```python
from build123d import *

# Parameters (mm, degrees)
SKETCH1_R           = 2.54
SKETCH1_R_2         = 2.25
BOSS_EXTRUDE1_DEPTH = 1.5875


with BuildPart() as part:
    # Sketch1 → Boss-Extrude1 (new body)
    with BuildSketch(Plane.XY):
        with BuildLine():
            Line((0, 0), (-44.45, 0))
            ThreePointArc((-44.45, 0), (-49.830627072, 1.070273269), (-54.392102448, 4.118153673))
            Line((-54.392102448, 4.118153673), (-86.142102448, 35.868153673))
            ThreePointArc((-86.142102448, 35.868153673), (-88.614208366, 37.519962038), (-91.530256121, 38.1))
            Line((-91.530256121, 38.1), (-99.06, 38.1))
            ThreePointArc((-99.06, 38.1), (-102.652102448, 36.612102448), (-104.14, 33.02))
            Line((-104.14, 33.02), (-104.14, 11.43))
            ThreePointArc((-104.14, 11.43), (-102.652102448, 7.837897552), (-99.06, 6.35))
            Line((-99.06, 6.35), (-99.06, -19.05))
            ThreePointArc((-99.06, -19.05), (-102.741703947, -21.834795846), (-104.14, -26.234204897))
            Line((-104.14, -26.234204897), (-104.14, -43.199318572))
            ThreePointArc((-104.14, -43.199318572), (-99.814124397, -51.831543955), (-90.309725681, -53.532990354))
            Line((-90.309725681, -53.532990354), (-38.1, -38.1))
            Line((-38.1, -38.1), (0, -38.1))
            Line((0, -38.1), (0, 0))
        make_face()
        with Locations((-89, 25.555)):
            Circle(SKETCH1_R, mode=Mode.SUBTRACT)
        with Locations((-89, -45.055)):
            Circle(SKETCH1_R, mode=Mode.SUBTRACT)
        with Locations((-18.24, -9.75)):
            Circle(SKETCH1_R, mode=Mode.SUBTRACT)
        with Locations((-74.5, -9.75)):
            Circle(SKETCH1_R_2, mode=Mode.SUBTRACT)
        with Locations((-48.5, -9.75)):
            Circle(SKETCH1_R_2, mode=Mode.SUBTRACT)
    extrude(amount=BOSS_EXTRUDE1_DEPTH)


solid = part.part
```
Build history of the part. All positions in model axes, mm. A direction names the side the tool comes from. Coordinates: 2 decimals unless noted, no trailing zeros. Order: outer loops, then holes, each group sorted by start corner. A loop starts at its lowest first (then second) coordinate and runs counter-clockwise, first axis right, second up. Notation, with made-up numbers: (-30.5, 0) -> (-15.5, 0) arc R32 ccw to (-15.5, 27) -> close; hole circle Ø5 at (4.5, 22). An arc over 180 degrees is marked (long way). Answer in a Markdown table with one row per item. Add a question column.
Q1. Drop flat-ended pins along their axis: pin 1 (3.5 mm diameter, centred on x = -74.5, y = -9.75, fed in from +Z); pin 2 (0.8 mm diameter, centred on x = -27, z = 1, fed in from +Y); pin 3 (0.5 mm diameter, centred on y = -11.5, z = 1, fed in from -X). Give the stop position or say it passes through.
Q2. Band-saw the part on A-A, the plane x = -89. List the corners of the cut face in (y, z) (1 decimal), then the cut area to 3 significant figures.
Q3. Mould opens along Y. For faces 3 (the face through (-88.576, 37.504, 0.783)), 4 (the face through (-17.068, -12.003, 0.783)), 5 (the face through (-64, -18, 0)) say: +Y half, -Y half, draft (parallel to the pull), parting line (faces both ways), or undercut.
Q4. Wall check: line 1 along Y through (x, z) = (-35, 0.15); line 2 along Y through (x, z) = (-48.5, 0.55); line 3 along Y through (x, z) = (-18.24, 0.75). Give the ranges that are in metal, low to high. Write a range as [from, to].
Q5. Band-saw the part on C-C, the plane x = -18.24. List the corners of the cut face in (y, z).
Q6. Which spindle directions (+Z, -Z, +X, -X, +Y, -Y) get a long thin tool onto all of the face, cutting with end or side? Do faces 1 (the face through (-102.612, 36.651, 0.783)), 2 (the face through (-102.691, 7.878, 0.783)). Say none if no direction does.
Q7. Band-saw the part on B-B, the plane y = -9.75. List the corners of the cut face in (x, z).
Q8. Band-saw the part on D-D, the plane z = 1.05. List the corners of the cut face in (x, y) (3 decimals).
Answers follow:
| question | item | result |
|---|---|---|
| 1 | pin 1 | through |
| 1 | pin 2 | y = 0 |
| 1 | pin 3 | x = -99.06 |
| 2 | outline | (-53.1, 0) -> (-47.6, 0) -> (-47.6, 1.6) -> (-53.1, 1.6) -> close; (-42.5, 0) -> (23, 0) -> (23, 1.6) -> (-42.5, 1.6) -> close; (28.1, 0) -> (37.7, 0) -> (37.7, 1.6) -> (28.1, 1.6) -> close |
| 2 | area | 128 mm^2 |
| 3 | face 3 | +Y half |
| 3 | face 4 | undercut |
| 3 | face 5 | draft |
| 4 | line 1 | [-38.1, 0] |
| 4 | line 2 | [-41.17, -12], [-7.5, 0.6] |
| 4 | line 3 | [-38.1, -12.29], [-7.21, 0] |
| 5 | outline | (-38.1, 0) -> (-12.29, 0) -> (-12.29, 1.59) -> (-38.1, 1.59) -> close; (-7.21, 0) -> (0, 0) -> (0, 1.59) -> (-7.21, 1.59) -> close |
| 6 | face 1 | +Z, -Z, -X, +Y |
| 6 | face 2 | +Z, -Z, -X |
| 7 | outline | (-99.06, 0) -> (-76.75, 0) -> (-76.75, 1.59) -> (-99.06, 1.59) -> close; (-72.25, 0) -> (-50.75, 0) -> (-50.75, 1.59) -> (-72.25, 1.59) -> close; (-46.25, 0) -> (-20.78, 0) -> (-20.78, 1.59) -> (-46.25, 1.59) -> close; (-15.7, 0) -> (0, 0) -> (0, 1.59) -> (-15.7, 1.59) -> close |
| 8 | outline | (-104.14, -43.199) arc R10.776 ccw to (-90.31, -53.533) -> (-38.1, -38.1) -> (0, -38.1) -> (0, 0) -> (-44.45, 0) arc R14.06 cw to (-54.392, 4.118) -> (-86.142, 35.868) arc R7.62 ccw to (-91.53, 38.1) -> (-99.06, 38.1) arc R5.08 ccw to (-104.14, 33.02) -> (-104.14, 11.43) arc R5.08 ccw to (-99.06, 6.35) -> (-99.06, -19.05) arc R7.62 ccw to (-104.14, -26.234) -> close; hole circle Ø5.08 at (-89, -45.055); hole circle Ø5.08 at (-89, 25.555); hole circle Ø4.5 at (-74.5, -9.75); hole circle Ø4.5 at (-48.5, -9.75); hole circle Ø5.08 at (-18.24, -9.75) |
